from build123d import *

# Parameters (mm, degrees)
SKETCH1_W           = 679.45
SKETCH1_H           = 1885.95
BOSS_EXTRUDE1_DEPTH = 11.43
SKETCH3_W           = 638.81
SKETCH3_H           = 1845.31
CUT_EXTRUDE2_DEPTH  = 1003.369977179
FILLET1_R           = 31.75
FILLET2_R           = 22.86


with BuildPart() as part:
    # Sketch1 → Boss-Extrude1 (new body)
    with BuildSketch(Plane(origin=(0, 0, 0), x_dir=(1, 0, 0), z_dir=(0, 1, 0))):
        Rectangle(SKETCH1_W, SKETCH1_H)
    extrude(amount=BOSS_EXTRUDE1_DEPTH)

    # Sketch3 → Cut-Extrude2 (cut, through all)
    with BuildSketch(Plane(origin=(0, 11.43, 0), x_dir=(1, 0, 0), z_dir=(0, 1, 0))):
        Rectangle(SKETCH3_W, SKETCH3_H)
    extrude(amount=-CUT_EXTRUDE2_DEPTH, mode=Mode.SUBTRACT)

    # Fillet1
    fillet1_edges = [part.edges().sort_by_distance(p)[0] for p in [
        (-339.725, 5.715, -942.975),
        (339.725, 5.715, -942.975),
        (339.725, 5.715, 942.975),
        (-339.725, 5.715, 942.975),
    ]]
    fillet(fillet1_edges, radius=FILLET1_R)

    # Fillet2
    fillet2_edges = [part.edges().sort_by_distance(p)[0] for p in [
        (-319.405, 5.715, -922.655),
        (319.405, 5.715, -922.655),
        (319.405, 5.715, 922.655),
        (-319.405, 5.715, 922.655),
    ]]
    fillet(fillet2_edges, radius=FILLET2_R)


solid = part.part
Design review of the part built by this model. Coordinates are the model's own, in mm. Coordinates: 2 decimals unless noted, no trailing zeros. Write each loop counter-clockwise with the first axis right and the second up, starting at its lowest first coordinate (ties: lowest second). Pieces come first, ordered by that corner, then holes. Notation, with made-up numbers: (19, 19) - (61, 19) arc R19 ccw to (61, 34) - close; hole circle Ø5 at (-6, -8.5). An arc over 180 degrees is marked (long way). One line per item, written item: value.
1) To check wall thickness, follow probe 1 along Z at (x, y) = (-269, 1.5) (3 decimals); probe 2 along X at (y, z) = (9.75, 132) (3 decimals); probe 3 along Z at (x, y) = (308.5, 6.5). State the ranges of each line that lie inside material, in increasing order.
Answer sheet:
probe 1: z = -942.975 to -922.655, 922.655 to 942.975
probe 2: x = -339.725 to -319.405, 319.405 to 339.725
probe 3: z = -942.97 to -919.28, 919.28 to 942.97
2) Add section C-C (y = 6). State the section outline as (x, z) points (3 decimals).
Answer sheet:
outline: (-339.725, -911.225) arc R31.75 ccw to (-307.975, -942.975) - (307.975, -942.975) arc R31.75 ccw to (339.725, -911.225) - (339.725, 911.225) arc R31.75 ccw to (307.975, 942.975) - (-307.975, 942.975) arc R31.75 ccw to (-339.725, 911.225) - close; hole (-319.405, -899.795) arc R22.86 ccw to (-296.545, -922.655) - (296.545, -922.655) arc R22.86 ccw to (319.405, -899.795) - (319.405, 899.795) arc R22.86 ccw to (296.545, 922.655) - (-296.545, 922.655) arc R22.86 ccw to (-319.405, 899.795) - close
3) Add section A-A (z = -601). State the section outline as (x, y) points (3 decimals), plus the area to 3 significant figures.
Answer sheet:
outline: (-339.725, 0) - (-319.405, 0) - (-319.405, 11.43) - (-339.725, 11.43) - close; (319.405, 0) - (339.725, 0) - (339.725, 11.43) - (319.405, 11.43) - close
area: 465 mm2
4) Add section B-B (x = -115.5). State the section outline as (y, z) points (3 decimals), plus the area to 3 significant figures.
Answer sheet:
outline: (0, -942.975) - (11.43, -942.975) - (11.43, -922.655) - (0, -922.655) - close; (0, 922.655) - (11.43, 922.655) - (11.43, 942.975) - (0, 942.975) - close
area: 465 mm2
